The model under review builds one solid part; all positions refer to its coordinate system, in mm. A direction names the side the tool comes from. Give positions to 0.01 mm unless a question says otherwise; leave off trailing zeros. Order: outer loops, then holes, each group sorted by start corner. A loop starts at its lowest first (then second) coordinate and runs counter-clockwise, first axis right, second up. Notation, with made-up numbers: M 28.25,-34 L 40.25,-34 A31 ccw 40.25,-1 Z; hole C 34,-4.75 d5. An arc over 180 degrees is marked long. One line per question, with ' | ' between items. Start each with the question number.
1. For faces 3 (the face through (0, -1.8, 2)), 4 (the face through (-0.97, -0.03, -1.27)), list the 3-axis set-ups (+Z, -Z, +X, -X, +Y, -Y) from which the entire face can be reached by the end or side of a thin tool; tool diameter is ignored.
2. We need section D-D on y = -1.5. Write out the cut boundary in (x, z), then the cut area to 3 significant figures.
3. Wall thickness on L1, parallel to X at y = -0.45, z = 0; L2, parallel to Y at x = -1.25, z = 3.5; L3, parallel to X at y = -0.1, z = -1.25: over which ranges is each line inside the solid? List them lowest first.
4. The part is to be moulded in two halves that separate along Z. For faces 1 (the face through (0, 1.8, 2)), 2 (the face through (-4.88, 0.01, -1.08)), say which applies: +Z half, -Z half, draft (parallel to the pull), parting line (faces both ways), or undercut.
5. Insertion check: P1, Ø2.5, axis at x = -1, z = 0.5, coming from the -Y side; P2, Ø2.5, axis at x = -1, z = 0, coming from the +Y side; P3, Ø2, axis at y = 0, z = 2, coming from the -X side; P4, Ø4, axis at x = 1, z = 2, coming from the +Y side. Each pin has a flat end and moves straight along its axis. Give the tip position at first contact, or say it passes through.
6. We need section C-C on y = -0.6. Write out the cut boundary in (x, z).
```python
from build123d import *

# Parameters (mm, degrees)
SKETCH_1_R      = 4
SKETCH_1_R_2    = 1.6
EXTRUDE_1_DEPTH = 1.8
SKETCH_2_R      = 5
SKETCH_2_R_2    = 4
EXTRUDE_2_DEPTH = 2
FILLET_1_R      = 1


with BuildPart() as part:
    # 草图1 → 凸台-拉伸1 (new, symmetric)
    with BuildSketch(Plane(origin=(0, 0, 0), x_dir=(1, 0, 0), z_dir=(0, 1, 0))):
        with Locations(Location((0, 0, 0), (0, 0, 270))):
            Circle(SKETCH_1_R)
        with Locations(Location((0, 0, 0), (0, 0, 270))):
            Circle(SKETCH_1_R_2, mode=Mode.SUBTRACT)
    extrude(amount=EXTRUDE_1_DEPTH, both=True)

    # 草图2 → 凸台-拉伸2 (add, symmetric)
    with BuildSketch(Plane(origin=(0, 0, 0), x_dir=(1, 0, 0), z_dir=(0, 1, 0))):
        with Locations(Location((0, 0, 0), (0, 0, 270))):
            Circle(SKETCH_2_R)
        with Locations(Location((0, 0, 0), (0, 0, 270))):
            Circle(SKETCH_2_R_2, mode=Mode.SUBTRACT)
    extrude(amount=EXTRUDE_2_DEPTH, both=True)

    # 圆角1
    fillet_1_edges = [part.edges().sort_by_distance(p)[0] for p in [
        (0, -2, -5),
        (0, 2, -5),
    ]]
    fillet(fillet_1_edges, radius=FILLET_1_R - 0.0001)  # a hair under: the kernel refuses the full size


solid = part.part
```
Entries:
1) face 3: -Y | face 4: +Y, -Y
2) outline: C 0,0 d9.73; hole C 0,0 d3.2 | area: 66.3 mm^2
3) L1: x = -5 to -1.6, 1.6 to 5 | L2: y = -1.8 to 1.8 | L3: x = -4.84 to -1, 1 to 4.84
4) face 1: undercut | face 2: parting line
5) P1: stops at y = -1.8 | P2: stops at y = 1.8 | P3: stops at x = -4.9 | P4: stops at y = 2
6) outline: C 0,0 d10; hole C 0,0 d3.2
